Check sheet for the modelled part. Datum: model origin and axes. Units: mm. Face numbers are marked on the shaded views. A direction names the side the tool comes from. Give positions to 0.01 mm unless a question says otherwise; leave off trailing zeros. Loops run counter-clockwise (first coordinate to the right, second up) from the corner with the lowest first, then second, coordinate; pieces in that order, holes last. Notation, with made-up numbers: (-30.75, 30) - (-4.75, 30) arc R28 ccw to (-4.75, 67) - close; hole circle Ø10 at (75.25, -9.75). An arc over 180 degrees is marked (long way). Use CSV: the item, a comma, the result in double quotes.
Autodesk Inventor part; units mm, degrees
ref_plane "YZ Plane" through (0, 0, 0) normal (1, 0, 0) x (0, 1, 0)
ref_plane "XZ Plane" through (0, 0, 0) normal (0, 1, 0) x (-1, 0, 0)
ref_plane "XY Plane" through (0, 0, 0) normal (0, 0, 1) x (1, 0, 0)
sketch "Esquisse1" plane through (0, 0, 0) normal (1, 0, 0) x (0, 1, 0)
  line L0 (0, 0) -> (25, 0)
  line L1 (25, 0) -> (25, -30)
  line L2 (25, -30) -> (0, -30)
  line L3 (0, -30) -> (0, 0)
  dimension "d0" = 25
  dimension "d1" = 30
extrude "Extrusion1" add sketch "Esquisse1" along normal blind 135
sketch "Esquisse2" plane through (0, 25, 0) normal (0, 1, 0) x (1, 0, 0)
  circle A0 centre (15, 15) radius 1.5
  line L0 (0, 30) -> (135, 30)
  line L1 (0, 30) -> (0, 0)
  circle A1 centre (120, 15) radius 1.5
  line L2 (135, 30) -> (135, 0)
  dimension "d4" = 3
  dimension "d5" = 15
  dimension "d6" = 15
  dimension "d7" = 3
  dimension "d9" = 15
extrude "Extrusion2" cut sketch "Esquisse2" against normal through all
sketch "Esquisse3" plane through (0, 0, 0) normal (0, 0, 1) x (1, 0, 0)
  line L0 (0, 25) -> (135, 25)
  line L1 (0, 25) -> (40, 25)
  line L2 (40, 25) -> (40, 12.5)
  line L3 (40, 12.5) -> (0, 12.5)
  line L4 (0, 12.5) -> (0, 25)
  line L5 (0, 0) -> (135, 0)
  line L6 (135, 0) -> (95, 0)
  line L7 (95, 0) -> (95, 12.5)
  line L8 (95, 12.5) -> (135, 12.5)
  line L9 (135, 12.5) -> (135, 0)
  dimension "d12" = 40
  dimension "d13" = 12.5
  dimension "d14" = 40
extrude "Extrusion3" cut sketch "Esquisse3" against normal through all
properties part number "entremoteur"
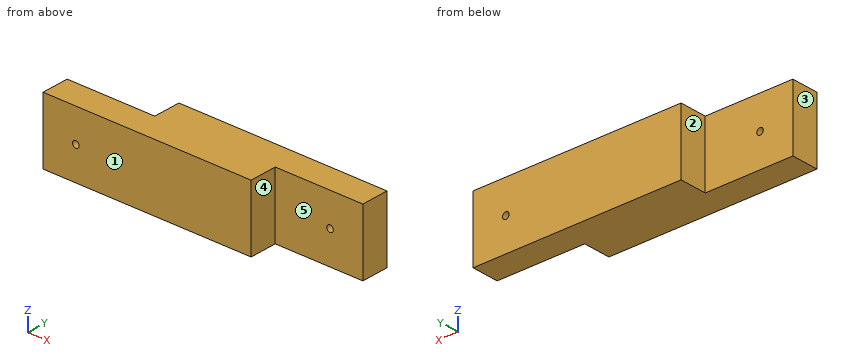
1. Sectioned sample at B-B, the plane z = -15. Record the boundary of the cut face in (x, y), and give its area (3 significant figures).
Completed:
outline,"(0, 0) - (13.5, 0) - (13.5, 12.5) - (0, 12.5) - close; (16.5, 0) - (95, 0) - (95, 12.5) - (118.5, 12.5) - (118.5, 25) - (40, 25) - (40, 12.5) - (16.5, 12.5) - close; (121.5, 12.5) - (135, 12.5) - (135, 25) - (121.5, 25) - close"
area,"2,300 mm²"
2. Sectioned sample at D-D, the plane y = 18.5. Record the boundary of the cut face in (x, z), and give its area (3 significant figures).
Completed:
outline,"(40, -30) - (135, -30) - (135, 0) - (40, 0) - close; hole circle Ø3 at (120, -15)"
area,"2,840 mm²"
3. Release check for a two-part mould opening along X. For the marked faces 3, 4 and 5 record: released by +X, released by -X, zero draft, split by the parting line, or undercut.
Completed:
face 3,"released by -X"
face 4,"released by +X"
face 5,"zero draft"
4. Sectioned sample at C-C, the plane z = -22. Record the boundary of the cut face in (x, y).
Completed:
outline,"(0, 0) - (95, 0) - (95, 12.5) - (135, 12.5) - (135, 25) - (40, 25) - (40, 12.5) - (0, 12.5) - close"
5. Set-up check for the marked faces 1 and 2: record each of +Z, -Z, +X, -X, +Y, -Y from which the full face is reachable in a straight line by a thin tool's end or side.
Completed:
face 1,"+Z, -Z, +X, -X, -Y"
face 2,"+Z, -Z, -X, +Y"
6. Scan lines: line 1 along X through (y, z) = (7, -15); line 2 along X through (y, z) = (21.75, -15); line 3 along Z through (x, y) = (120, 16.75). Record each from-to range of solid material in increasing order.
Completed:
line 1,"x = 0 to 13.5, 16.5 to 95"
line 2,"x = 40 to 118.5, 121.5 to 135"
line 3,"z = -30 to -16.5, -13.5 to 0"
7. Sectioned sample at A-A, the plane x = 15. Record the boundary of the cut face in (y, z).
Completed:
outline,"(0, -30) - (12.5, -30) - (12.5, -16.5) - (0, -16.5) - close; (0, -13.5) - (12.5, -13.5) - (12.5, 0) - (0, 0) - close"
8. Go/stop test with a flat-tipped pin: pin 1 Ø15 at (x, z) = (114, -8.5) entering from -Y. Record where the tip stops, or that it passes through.
Completed:
pin 1,"stops at y = 12.5"
